Geometry: see drawing. Coordinates: mm, zero at the bounding-box minimum. Give positions to 0.01 mm unless a question says otherwise; leave off trailing zeros. Order: outer loops, then holes, each group sorted by start corner. A loop starts at its lowest first (then second) coordinate and runs counter-clockwise, first axis right, second up. Notation, with made-up numbers: (38.5, 69.25) - (97.5, 69.25) arc R21 ccw to (97.5, 106.25) - close; hole circle Ø2 at (-6.5, 87). An arc over 180 degrees is marked (long way). Put each result on its own line as item: value. Start each with the question number.
1. Section B-B on x = 66.04. Return the cut outline in (y, z), plus the area to 3 significant figures.
2. Ray query, line 1 along Y through (x, z) = (15.24, 1.65); line 2 along Y through (x, z) = (66.04, 1); line 3 along X through (y, z) = (14.5, 1.9). Return the intervals inside material, ascending. Write a range as from..to.
3. Section A-A on y = 9.2. Return the cut outline in (x, z), plus the area to 3 significant figures.
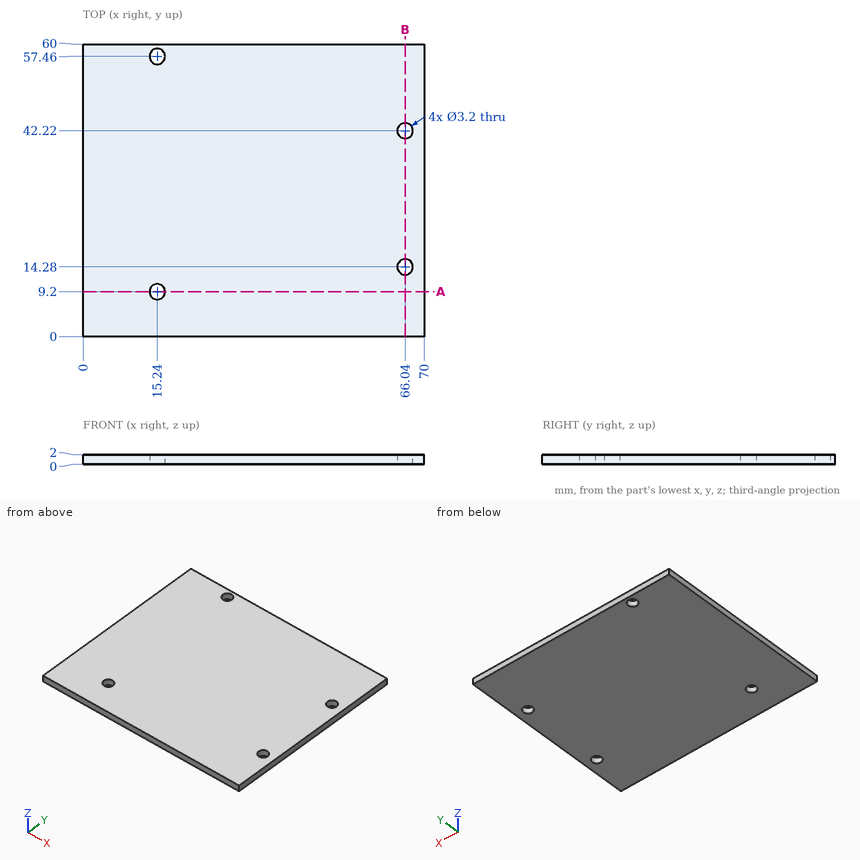
Resolved:
1. outline: (0, 0) - (12.68, 0) - (12.68, 2) - (0, 2) - close; (15.88, 0) - (40.62, 0) - (40.62, 2) - (15.88, 2) - close; (43.82, 0) - (60, 0) - (60, 2) - (43.82, 2) - close
1. area: 107 mm^2
2. line 1: 0..7.6, 10.8..55.86, 59.06..60
2. line 2: 0..12.68, 15.88..40.62, 43.82..60
2. line 3: 0..64.46, 67.62..70
3. outline: (0, 0) - (13.64, 0) - (13.64, 2) - (0, 2) - close; (16.84, 0) - (70, 0) - (70, 2) - (16.84, 2) - close
3. area: 134 mm^2
